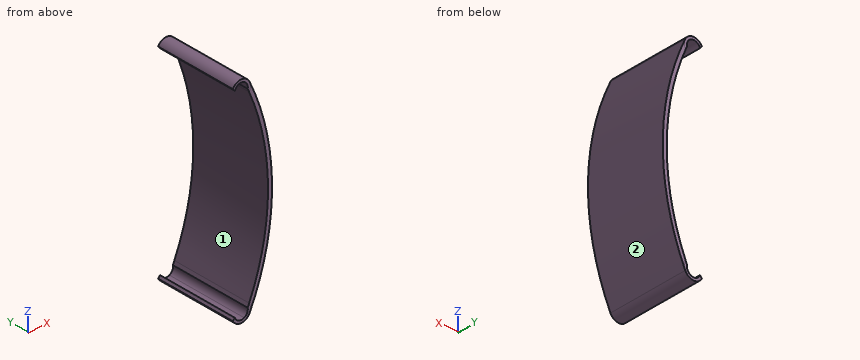
Autodesk Inventor part; units mm, degrees
ref_plane "YZ Plane" through (0, 0, 0) normal (1, 0, 0) x (0, 1, 0)
ref_plane "XZ Plane" through (0, 0, 0) normal (0, 1, 0) x (-1, 0, 0)
ref_plane "XY Plane" through (0, 0, 0) normal (0, 0, 1) x (1, 0, 0)
sketch "スケッチ1" plane through (0, 0, 0) normal (0, 1, 0) x (-1, 0, 0)
  arc A0 (8.4334, 37.592) -> (8.4334, -37.592) centre (88, 0) ccw
  arc A1 (8.5926, 34.3032) -> (8.5926, -34.3032) centre (88, 0) ccw
  line L0 (0, -123.2) -> (0, 123.2) construction
  line L1 (211.2, 0) -> (-35.2, 0) construction
  line L2 (88, 0) -> (38.8561, -49.1439)
  line L3 (88, 0) -> (38.8561, 49.1439)
  circle A2 centre (88, 0) radius 88 construction
  line L4 (38.8561, -49.1439) -> (21.1784, -31.4663) construction
  line L5 (21.1784, -31.4663) -> (10.6608, -41.9839) construction
  line L6 (38.8561, 49.1439) -> (21.1784, 31.4663) construction
  line L7 (21.1784, 31.4663) -> (10.6608, 41.9839) construction
  circle A3 centre (11.598, 36.0969) radius 3.5
  circle A4 centre (11.598, 36.0969) radius 2.5
  circle A5 centre (11.598, -36.0969) radius 3.5
  circle A6 centre (11.598, -36.0969) radius 2.5
  arc A7 (14.7014, 37.7152) -> (12.2579, 32.6597) centre (21.1784, 31.4663) ccw
  arc A8 (12.2579, -32.6597) -> (14.7014, -37.7152) centre (21.1784, -31.4663) ccw
  arc A9 (9.1534, 35.5734) -> (10.45, -38.3177) centre (88, 0) ccw
  point P0 (0, 0)
  point P1 (12.4744, 33.7556)
  point P2 (13.9772, 36.8646)
  point P3 (8.4334, -37.592)
  point P4 (14.7014, -37.7152)
  point P5 (13.9772, -36.8646)
  point P6 (12.4744, -33.7556)
  point P7 (12.2579, -32.6597)
  point P8 (8.5926, -34.3032)
  point P9 (8.5926, 34.3032)
  point P10 (9.1534, -35.5734)
  point P11 (8.5926, -34.3032)
  dimension "d6" = 5
  dimension "d0" = 88
  dimension "d2" = 86.5
  dimension "d3" = 69.5
  dimension "d4" = 176
  dimension "d5" = 25
  dimension "d7" = 7
  dimension "d8" = 9
extrude "押し出し1" add sketch "スケッチ1" along normal blind 31 contours A3 A1 A5 A0 | A3 A7 A4 A9 | A5 A9 A6 A8 picked at (10.6807, 39.1053) picked at (8.9829, -37.8462)
properties part number "Machine_Cover"
Work out the finished part from the listing and answer in its coordinate system (mm). Face numbers are marked on the shaded views. Coordinates: 2 decimals unless noted, no trailing zeros. Write each loop counter-clockwise with the first axis right and the second up, starting at its lowest first coordinate (ties: lowest second). Pieces come first, ordered by that corner, then holes. Notation, with made-up numbers: M -39.5,60.5 L -35.5,60.5 A17 ccw -35.5,78.5 Z; hole C 72,35.5 d6. An arc over 180 degrees is marked long. Use one line per item in the form item = value. Start each with the question number.
1. The part is cut by section C-C (x = -2.75). Give the vertices of the cut face in (y, z), plus the area to 3 significant figures.
2. The part is cut by section B-B (y = 9). Give the vertices of the cut face in (x, z).
3. Straight lines are drawn through the part: probe 1 along Z at (x, y) = (-13, 25.5); probe 2 along Z at (x, y) = (-10.5, 21.5); probe 3 along X at (y, z) = (4, 14). For each, find the intervals that lie inside material, in ascending order. Write a range as from..to.
4. The mould has two halves that part along Z. Classify the marked faces 1 and 2: released by +Z, released by -Z, zero draft, split by the parting line, or undercut.
5. Each of these flat-tipped pins is pushed along its axis until it touches: P1, Ø2, axis at y = 26, z = 21, coming from the -X side; P2, Ø1, axis at x = -3, z = -3.5, coming from the -Y side; P3, Ø1.5, axis at y = 15.5, z = -31.5, coming from the -X side; P4, Ø5, axis at y = 8.5, z = -31.5, coming from the -X side. Where does it stop, or does it pass through?
6. The part is cut by section A-A (x = -11.75). Give the vertices of the cut face in (y, z).
Evaluation:
q1.outline = M 0,-21.83 L 31,-21.83 L 31,-14.65 L 0,-14.65 Z; M 0,14.65 L 31,14.65 L 31,21.83 L 0,21.83 Z
q1.area = 445 mm^2
q2.outline = M -14.7,-37.72 A3.5 ccw -8.43,-37.59 A88 ccw -8.43,37.59 A3.5 ccw -14.7,37.72 A9 cw -13.98,36.86 A2.5 cw -9.15,35.57 A86.5 cw -8.59,34.3 A86.5 cw -8.59,-34.3 A86.5 cw -9.15,-35.57 A2.5 cw -13.98,-36.86 A9 cw Z
q3.probe_1 = -39.3..-38.17, 38.17..39.3
q3.probe_2 = -39.42..-38.34, 38.34..39.42
q3.probe_3 = -2.64..-1.12
q4.face_1 = undercut
q4.face_2 = split by the parting line
q5.P1 = -4.34
q5.P2 = through
q5.P3 = -7.74
q5.P4 = -8.46
q6.outline = M 0,-39.59 L 31,-39.59 L 31,-38.59 L 0,-38.59 Z; M 0,38.59 L 31,38.59 L 31,39.59 L 0,39.59 Z
